Verification items for the finished model (mm, model axes). A direction names the side the tool comes from. Give positions to 0.01 mm unless a question says otherwise; leave off trailing zeros. Order: outer loops, then holes, each group sorted by start corner. A loop starts at its lowest first (then second) coordinate and runs counter-clockwise, first axis right, second up. Notation, with made-up numbers: (10.25, 63) -> (19.25, 63) arc R37 ccw to (19.25, 99) -> close; hole circle Ø1 at (71, -2.75). An arc over 180 degrees is marked (long way). One line per question, with ' | ' between items. Start each with the question number.
Q1. Section check C-C on y = 21. Record the cut outline in (x, z).
Q2. Go/stop test with flat-tipped pins: pin 1 (1.5 mm diameter, centred on x = 16, y = 19.5, fed in from -Z); pin 2 (2 mm diameter, centred on x = 11.15, y = 21.25, fed in from -Z); pin 3 (6 mm diameter, centred on y = 10.5, z = -0.5, fed in from -X). Record where each tip stops, or that it passes through.
Q3. Section check D-D on x = 13.5. Record the cut outline in (y, z), plus the area to 3 significant figures.
Q4. Section check B-B on x = -12. Record the cut outline in (y, z), plus the area to 3 significant figures.
Q5. Material ranges on probe 1 along Y at (x, z) = (8.5, -7.25); probe 2 along Z at (x, y) = (14, 1); probe 3 along X at (y, z) = (6.5, -11.5), recorded low to high. Write a range as [from, to].
Q6. Section check A-A on y = -1.5. Record the cut outline in (x, z).
Q7. Mould release check, pull along X, two halves, no side actions. Record for faces 3 (the flat face through (7, 5, 0)), 4 (the cylindrical face through (10.966, 7.416, -6.409)), 5 (the flat face through (0, 0, 2)): released by +X, released by -X, zero draft, split by the parting line, or undercut.
Q8. Access from +Z, -Z, +X, -X, +Y, -Y to the whole of each face (thin tool, end or side, straight path). Record for faces 1 (the cylindrical face through (25.64, 1.34, 0.99)), 2 (the cylindrical face through (5.01, 3.93, -5.92)).
Autodesk Inventor part; units mm, degrees
ref_plane "YZ Plane" through (0, 0, 0) normal (1, 0, 0) x (0, 1, 0)
ref_plane "XZ Plane" through (0, 0, 0) normal (0, 1, 0) x (-1, 0, 0)
ref_plane "XY Plane" through (0, 0, 0) normal (0, 0, 1) x (1, 0, 0)
sketch "Sketch2" plane through (0, 0, 0) normal (0, 0, 1) x (1, 0, 0)
  circle A0 centre (0, 0) radius 26.5
  dimension "d0" = 53
extrude "Extrusion1" add sketch "Sketch2" along normal blind 2
sketch "Sketch3" plane through (0, 0, 2) normal (0, 0, 1) x (1, 0, 0)
  circle A0 centre (-12.8301, 20.2827) radius 1.2295 construction
  circle A1 centre (-11.1503, -21.2526) radius 1.2295 construction
  circle A2 centre (23.9804, 0.9699) radius 1.2295 construction
  circle A3 centre (12.8301, -20.2827) radius 1.2295 construction
  circle A4 centre (-23.9804, -0.9699) radius 1.2295 construction
  circle A5 centre (11.1503, 21.2526) radius 1.2295 construction
  circle A6 centre (0, 0) radius 26.5 construction
  circle A7 centre (0, 0) radius 21.5
  point P0 (0, 0)
hole "Hole1" at (23.9804, 0.9699, 2) at (12.8301, -20.2827, 2) at (-11.1503, -21.2526, 2) at (-23.9804, -0.9699, 2) at (-12.8301, 20.2827, 2) at (11.1503, 21.2526, 2) direction (0, 0, -1) diameter 3.4 end through all
sketch "Sketch4" plane through (0, 0, 0) normal (0, 0, -1) x (-1, 0, 0)
  circle A0 centre (-7.3947, 4.6777) radius 2.5
  circle A1 centre (-7.3947, 4.6777) radius 4.5
  circle A2 centre (-7.3947, 4.6777) radius 6 construction
  point P0 (0, 0)
  dimension "d10" = 5
  dimension "d11" = 2
extrude "Extrusion2" add sketch "Sketch4" along normal blind 13
chamfer "Chamfer1" distance 1 angle 45 1 edges at (9.8947, 4.6777, -13)
properties part number "P019" material "Aluminium"
Filled in:
1) outline: (-16.16, 0) -> (-14.37, 0) -> (-14.37, 2) -> (-16.16, 2) -> close; (-11.29, 0) -> (9.47, 0) -> (9.47, 2) -> (-11.29, 2) -> close; (12.83, 0) -> (16.16, 0) -> (16.16, 2) -> (12.83, 2) -> close
2) pin 1: z = 0 | pin 2: through | pin 3: x = -25.4
3) outline: (-22.8, 0) -> (-21.85, 0) -> (-21.85, 2) -> (-22.8, 2) -> close; (-18.72, 0) -> (22.8, 0) -> (22.8, 2) -> (-18.72, 2) -> close | area: 85.0 mm²
4) outline: (-23.63, 0) -> (-22.73, 0) -> (-22.73, 2) -> (-23.63, 2) -> close; (-19.78, 0) -> (18.8, 0) -> (18.8, 2) -> (-19.78, 2) -> close; (21.77, 0) -> (23.63, 0) -> (23.63, 2) -> (21.77, 2) -> close | area: 82.7 mm²
5) probe 1: [0.32, 2.44], [6.92, 9.04] | probe 2: [0, 2] | probe 3: [3.28, 5.68], [9.11, 11.51]
6) outline: (-26.46, 0) -> (-25.6, 0) -> (-25.6, 2) -> (-26.46, 2) -> close; (-22.37, 0) -> (26.46, 0) -> (26.46, 2) -> (-22.37, 2) -> close
7) face 3: undercut | face 4: split by the parting line | face 5: zero draft
8) face 1: +Z, -Z | face 2: -Z
